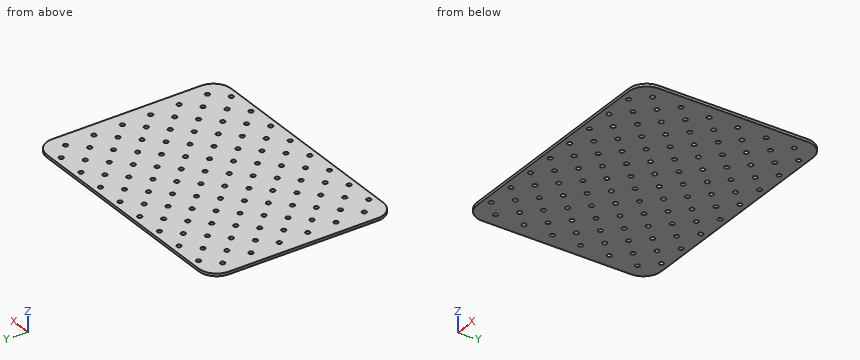
from build123d import *

# Parameters (mm, degrees)
PAD_DEPTH                        = 3
SKETCH001_R                      = 2.5
HOLE_DEPTH                       = 713.541639
SKETCH001_LINEARPATTERN_2_R      = 2.5
HOLE_LINEARPATTERN_2_DEPTH       = 713.541639
SKETCH001_LINEARPATTERN_3_R      = 2.5
HOLE_LINEARPATTERN_3_DEPTH       = 713.541639
SKETCH001_LINEARPATTERN_4_R      = 2.5
HOLE_LINEARPATTERN_4_DEPTH       = 713.541639
SKETCH001_LINEARPATTERN_5_R      = 2.5
HOLE_LINEARPATTERN_5_DEPTH       = 713.541639
SKETCH001_LINEARPATTERN_6_R      = 2.5
HOLE_LINEARPATTERN_6_DEPTH       = 713.541639
SKETCH001_LINEARPATTERN_7_R      = 2.5
HOLE_LINEARPATTERN_7_DEPTH       = 713.541639
SKETCH001_LINEARPATTERN_8_R      = 2.5
HOLE_LINEARPATTERN_8_DEPTH       = 713.541639
SKETCH001_LINEARPATTERN_9_R      = 2.5
HOLE_LINEARPATTERN_9_DEPTH       = 713.541639
LINEARPATTERN001_COUNT           = 6
LINEARPATTERN001_PITCH           = 32
SKETCH002_R                      = 2.5
HOLE001_DEPTH                    = 713.541639
SKETCH002_LINEARPATTERN002_2_R   = 2.5
HOLE001_LINEARPATTERN002_2_DEPTH = 713.541639
SKETCH002_LINEARPATTERN002_3_R   = 2.5
HOLE001_LINEARPATTERN002_3_DEPTH = 713.541639
SKETCH002_LINEARPATTERN002_4_R   = 2.5
HOLE001_LINEARPATTERN002_4_DEPTH = 713.541639
SKETCH002_LINEARPATTERN002_5_R   = 2.5
HOLE001_LINEARPATTERN002_5_DEPTH = 713.541639
SKETCH002_LINEARPATTERN002_6_R   = 2.5
HOLE001_LINEARPATTERN002_6_DEPTH = 713.541639
SKETCH002_LINEARPATTERN002_7_R   = 2.5
HOLE001_LINEARPATTERN002_7_DEPTH = 713.541639
SKETCH002_LINEARPATTERN002_8_R   = 2.5
HOLE001_LINEARPATTERN002_8_DEPTH = 713.541639
LINEARPATTERN003_COUNT           = 7
LINEARPATTERN003_PITCH           = 32


with BuildPart() as part:
    # Sketch → Pad (new body)
    with BuildSketch(Plane.XY):
        with BuildLine():
            Line((-124, 104), (124, 104))
            ThreePointArc((144, 84), (138.142136, 98.142136), (124, 104))
            Line((144, 84), (144, -84))
            ThreePointArc((124, -104), (138.142136, -98.142136), (144, -84))
            Line((124, -104), (-124, -104))
            ThreePointArc((-144, -84), (-138.142136, -98.142136), (-124, -104))
            Line((-144, -84), (-144, 84))
            ThreePointArc((-124, 104), (-138.142136, 98.142136), (-144, 84))
        make_face()
    extrude(amount=PAD_DEPTH)

    # Sketch001 → Hole (cut, through all)
    with BuildSketch(Plane.XY):
        with Locations((128, 80)):
            Circle(SKETCH001_R)
    hole = extrude(amount=HOLE_DEPTH, mode=Mode.SUBTRACT)

    # Sketch001 LinearPattern 2 → Hole LinearPattern 2 (cut, through all)
    with BuildSketch(Plane(origin=(-32, 0, 0), x_dir=(1, 0, 0), z_dir=(0, 0, 1))):
        with Locations((128, 80)):
            Circle(SKETCH001_LINEARPATTERN_2_R)
    hole_linearpattern_2 = extrude(amount=HOLE_LINEARPATTERN_2_DEPTH, mode=Mode.SUBTRACT)

    # Sketch001 LinearPattern 3 → Hole LinearPattern 3 (cut, through all)
    with BuildSketch(Plane(origin=(-64, 0, 0), x_dir=(1, 0, 0), z_dir=(0, 0, 1))):
        with Locations((128, 80)):
            Circle(SKETCH001_LINEARPATTERN_3_R)
    hole_linearpattern_3 = extrude(amount=HOLE_LINEARPATTERN_3_DEPTH, mode=Mode.SUBTRACT)

    # Sketch001 LinearPattern 4 → Hole LinearPattern 4 (cut, through all)
    with BuildSketch(Plane(origin=(-96, 0, 0), x_dir=(1, 0, 0), z_dir=(0, 0, 1))):
        with Locations((128, 80)):
            Circle(SKETCH001_LINEARPATTERN_4_R)
    hole_linearpattern_4 = extrude(amount=HOLE_LINEARPATTERN_4_DEPTH, mode=Mode.SUBTRACT)

    # Sketch001 LinearPattern 5 → Hole LinearPattern 5 (cut, through all)
    with BuildSketch(Plane(origin=(-128, 0, 0), x_dir=(1, 0, 0), z_dir=(0, 0, 1))):
        with Locations((128, 80)):
            Circle(SKETCH001_LINEARPATTERN_5_R)
    hole_linearpattern_5 = extrude(amount=HOLE_LINEARPATTERN_5_DEPTH, mode=Mode.SUBTRACT)

    # Sketch001 LinearPattern 6 → Hole LinearPattern 6 (cut, through all)
    with BuildSketch(Plane(origin=(-160, 0, 0), x_dir=(1, 0, 0), z_dir=(0, 0, 1))):
        with Locations((128, 80)):
            Circle(SKETCH001_LINEARPATTERN_6_R)
    hole_linearpattern_6 = extrude(amount=HOLE_LINEARPATTERN_6_DEPTH, mode=Mode.SUBTRACT)

    # Sketch001 LinearPattern 7 → Hole LinearPattern 7 (cut, through all)
    with BuildSketch(Plane(origin=(-192, 0, 0), x_dir=(1, 0, 0), z_dir=(0, 0, 1))):
        with Locations((128, 80)):
            Circle(SKETCH001_LINEARPATTERN_7_R)
    hole_linearpattern_7 = extrude(amount=HOLE_LINEARPATTERN_7_DEPTH, mode=Mode.SUBTRACT)

    # Sketch001 LinearPattern 8 → Hole LinearPattern 8 (cut, through all)
    with BuildSketch(Plane(origin=(-224, 0, 0), x_dir=(1, 0, 0), z_dir=(0, 0, 1))):
        with Locations((128, 80)):
            Circle(SKETCH001_LINEARPATTERN_8_R)
    hole_linearpattern_8 = extrude(amount=HOLE_LINEARPATTERN_8_DEPTH, mode=Mode.SUBTRACT)

    # Sketch001 LinearPattern 9 → Hole LinearPattern 9 (cut, through all)
    with BuildSketch(Plane(origin=(-256, 0, 0), x_dir=(1, 0, 0), z_dir=(0, 0, 1))):
        with Locations((128, 80)):
            Circle(SKETCH001_LINEARPATTERN_9_R)
    hole_linearpattern_9 = extrude(amount=HOLE_LINEARPATTERN_9_DEPTH, mode=Mode.SUBTRACT)

    # LinearPattern001: Hole, Hole LinearPattern 2, Hole LinearPattern 3, Hole LinearPattern 4, Hole LinearPattern 5, Hole LinearPattern 6, Hole LinearPattern 7, Hole LinearPattern 8, Hole LinearPattern 9 ×6
    with Locations(*[(0, -i * LINEARPATTERN001_PITCH, 0) for i in range(1, LINEARPATTERN001_COUNT)]):
        add(hole, mode=Mode.SUBTRACT)
        add(hole_linearpattern_2, mode=Mode.SUBTRACT)
        add(hole_linearpattern_3, mode=Mode.SUBTRACT)
        add(hole_linearpattern_4, mode=Mode.SUBTRACT)
        add(hole_linearpattern_5, mode=Mode.SUBTRACT)
        add(hole_linearpattern_6, mode=Mode.SUBTRACT)
        add(hole_linearpattern_7, mode=Mode.SUBTRACT)
        add(hole_linearpattern_8, mode=Mode.SUBTRACT)
        add(hole_linearpattern_9, mode=Mode.SUBTRACT)

    # Sketch002 → Hole001 (cut, through all)
    with BuildSketch(Plane.XY):
        with Locations((112, 96)):
            Circle(SKETCH002_R)
    hole001 = extrude(amount=HOLE001_DEPTH, mode=Mode.SUBTRACT)

    # Sketch002 LinearPattern002 2 → Hole001 LinearPattern002 2 (cut, through all)
    with BuildSketch(Plane(origin=(-32, 0, 0), x_dir=(1, 0, 0), z_dir=(0, 0, 1))):
        with Locations((112, 96)):
            Circle(SKETCH002_LINEARPATTERN002_2_R)
    hole001_linearpattern002_2 = extrude(amount=HOLE001_LINEARPATTERN002_2_DEPTH, mode=Mode.SUBTRACT)

    # Sketch002 LinearPattern002 3 → Hole001 LinearPattern002 3 (cut, through all)
    with BuildSketch(Plane(origin=(-64, 0, 0), x_dir=(1, 0, 0), z_dir=(0, 0, 1))):
        with Locations((112, 96)):
            Circle(SKETCH002_LINEARPATTERN002_3_R)
    hole001_linearpattern002_3 = extrude(amount=HOLE001_LINEARPATTERN002_3_DEPTH, mode=Mode.SUBTRACT)

    # Sketch002 LinearPattern002 4 → Hole001 LinearPattern002 4 (cut, through all)
    with BuildSketch(Plane(origin=(-96, 0, 0), x_dir=(1, 0, 0), z_dir=(0, 0, 1))):
        with Locations((112, 96)):
            Circle(SKETCH002_LINEARPATTERN002_4_R)
    hole001_linearpattern002_4 = extrude(amount=HOLE001_LINEARPATTERN002_4_DEPTH, mode=Mode.SUBTRACT)

    # Sketch002 LinearPattern002 5 → Hole001 LinearPattern002 5 (cut, through all)
    with BuildSketch(Plane(origin=(-128, 0, 0), x_dir=(1, 0, 0), z_dir=(0, 0, 1))):
        with Locations((112, 96)):
            Circle(SKETCH002_LINEARPATTERN002_5_R)
    hole001_linearpattern002_5 = extrude(amount=HOLE001_LINEARPATTERN002_5_DEPTH, mode=Mode.SUBTRACT)

    # Sketch002 LinearPattern002 6 → Hole001 LinearPattern002 6 (cut, through all)
    with BuildSketch(Plane(origin=(-160, 0, 0), x_dir=(1, 0, 0), z_dir=(0, 0, 1))):
        with Locations((112, 96)):
            Circle(SKETCH002_LINEARPATTERN002_6_R)
    hole001_linearpattern002_6 = extrude(amount=HOLE001_LINEARPATTERN002_6_DEPTH, mode=Mode.SUBTRACT)

    # Sketch002 LinearPattern002 7 → Hole001 LinearPattern002 7 (cut, through all)
    with BuildSketch(Plane(origin=(-192, 0, 0), x_dir=(1, 0, 0), z_dir=(0, 0, 1))):
        with Locations((112, 96)):
            Circle(SKETCH002_LINEARPATTERN002_7_R)
    hole001_linearpattern002_7 = extrude(amount=HOLE001_LINEARPATTERN002_7_DEPTH, mode=Mode.SUBTRACT)

    # Sketch002 LinearPattern002 8 → Hole001 LinearPattern002 8 (cut, through all)
    with BuildSketch(Plane(origin=(-224, 0, 0), x_dir=(1, 0, 0), z_dir=(0, 0, 1))):
        with Locations((112, 96)):
            Circle(SKETCH002_LINEARPATTERN002_8_R)
    hole001_linearpattern002_8 = extrude(amount=HOLE001_LINEARPATTERN002_8_DEPTH, mode=Mode.SUBTRACT)

    # LinearPattern003: Hole001, Hole001 LinearPattern002 2, Hole001 LinearPattern002 3, Hole001 LinearPattern002 4, Hole001 LinearPattern002 5, Hole001 LinearPattern002 6, Hole001 LinearPattern002 7, Hole001 LinearPattern002 8 ×7
    with Locations(*[(0, -i * LINEARPATTERN003_PITCH, 0) for i in range(1, LINEARPATTERN003_COUNT)]):
        add(hole001, mode=Mode.SUBTRACT)
        add(hole001_linearpattern002_2, mode=Mode.SUBTRACT)
        add(hole001_linearpattern002_3, mode=Mode.SUBTRACT)
        add(hole001_linearpattern002_4, mode=Mode.SUBTRACT)
        add(hole001_linearpattern002_5, mode=Mode.SUBTRACT)
        add(hole001_linearpattern002_6, mode=Mode.SUBTRACT)
        add(hole001_linearpattern002_7, mode=Mode.SUBTRACT)
        add(hole001_linearpattern002_8, mode=Mode.SUBTRACT)


solid = part.part
For this review, take the finished solid that the model builds, in its own axes (mm). Give positions to 0.01 mm unless a question says otherwise; leave off trailing zeros.
Item 1: For line 1 along X through (y, z) = (86.5, 0.9); line 2 along X through (y, z) = (91, 0.8) (3 decimals), list the stretches that pass through material, from the lowest coordinate up.
Item 2: Take a section at A-A, the plane z = 0.6. Give the number of separate pieces and of enclosed holes in the cut face, and give its area (3 significant figures).
Item 3: Insertion check: pin 1 (4.5 mm diameter, centred on x = -64, y = -16, fed in from -Z). The pin has a flat end and moves straight along its axis. Give the tip position at first contact, or say it passes through.
Calculated:
1. line 1: x = -143.84 to 143.84
1. line 2: x = -142.735 to 142.735
2. separate pieces: 1
2. enclosed holes: 110
2. area: 57,400 mm2
3. pin 1: passes through
